from build123d import *

# Parameters (mm, degrees)
AUFSATZ_LINEAR_AUSTRAGEN1_DEPTH    = 40
DURCHGANGSLOCH_F_R_M81_D           = 8.4
DURCHGANGSLOCH_F_R_M3_51_D         = 3.7
DURCHGANGSLOCH_F_R_M82_D           = 8.4
DURCHGANGSLOCH_F_R_M82_CSINK_D     = 8.45
DURCHGANGSLOCH_F_R_M82_CSINK_ANGLE = 90
SKIZZE21_R                         = 5
SCHNITT_LINEAR_AUSTRAGEN1_DEPTH    = 12
SKIZZE22_W                         = 70
SKIZZE22_H                         = 14.633500803
SCHNITT_LINEAR_AUSTRAGEN2_DEPTH    = 20
SKIZZE23_W                         = 70
SKIZZE23_H                         = 15
SCHNITT_LINEAR_AUSTRAGEN3_DEPTH    = 26
SKIZZE25_W                         = 70
SKIZZE25_H                         = 2
SCHNITT_LINEAR_AUSTRAGEN5_DEPTH    = 26
SCHNITT_LINEAR_AUSTRAGEN6_DEPTH    = 3


with BuildPart() as part:
    # Skizze1 → Aufsatz-Linear austragen1 (new body)
    with BuildSketch(Plane.XY):
        Polygon((-85.072105864, 34.368747103), (-85.072105864, 14.368747103), (-50.072105864, 14.368747103), (-50.072105864, 28.368747103), (-65.805439197, 28.368747103), (-65.805439197, 34.368747103), align=None)
        Polygon((-50.072105864, 28.368747103), (-50.072105864, 14.368747103), (-15.072105864, 14.368747103), (-15.072105864, 34.368747103), (-34.33877253, 34.368747103), (-34.33877253, 28.368747103), align=None)
    extrude(amount=AUFSATZ_LINEAR_AUSTRAGEN1_DEPTH)

    # Durchgangsloch für M81 (through all)
    with Locations(Plane(origin=(0, 34.368747103, 0), x_dir=(1, 0, 0), z_dir=(0, 1, 0))):
        with Locations((-78.072105864, -33), (-22.072105864, -33)):
            Hole(DURCHGANGSLOCH_F_R_M81_D / 2)

    # Durchgangsloch für M3.51 (through all)
    with Locations(Plane(origin=(0, 34.368747103, 0), x_dir=(1, 0, 0), z_dir=(0, 1, 0))):
        with Locations((-78.072105864, -5), (-78.072105864, -20), (-22.072105864, -20), (-22.072105864, -5)):
            Hole(DURCHGANGSLOCH_F_R_M3_51_D / 2)

    # Durchgangsloch für M82 (through all)
    with Locations(Plane(origin=(0, 14.368747103, 0), x_dir=(-1, 0, 0), z_dir=(0, -1, 0))):
        with Locations((50.072105864, -33)):
            CounterSinkHole(DURCHGANGSLOCH_F_R_M82_D / 2, DURCHGANGSLOCH_F_R_M82_CSINK_D / 2, counter_sink_angle=DURCHGANGSLOCH_F_R_M82_CSINK_ANGLE)

    # Skizze21 → Schnitt-Linear austragen1 (cut)
    with BuildSketch(Plane(origin=(0, 28.368747103, 0), x_dir=(1, 0, 0), z_dir=(0, 1, 0))):
        with Locations((-50.072105864, -33)):
            Circle(SKIZZE21_R)
    extrude(amount=-SCHNITT_LINEAR_AUSTRAGEN1_DEPTH, mode=Mode.SUBTRACT)

    # Skizze22 → Schnitt-Linear austragen2 (cut)
    with BuildSketch(Plane(origin=(0, 34.368747103, 0), x_dir=(1, 0, 0), z_dir=(0, 1, 0))):
        with Locations((-50.072105864, -32.683249598)):
            Rectangle(SKIZZE22_W, SKIZZE22_H)
    extrude(amount=-SCHNITT_LINEAR_AUSTRAGEN2_DEPTH, mode=Mode.SUBTRACT)

    # Skizze23 → Schnitt-Linear austragen3 (cut)
    with BuildSketch(Plane(origin=(0, 0, 0), x_dir=(-1, 0, 0), z_dir=(0, 0, -1))):
        with Locations((50.072105864, 26.868747103)):
            Rectangle(SKIZZE23_W, SKIZZE23_H)
    extrude(amount=-SCHNITT_LINEAR_AUSTRAGEN3_DEPTH, mode=Mode.SUBTRACT)

    # Skizze25 → Schnitt-Linear austragen5 (cut)
    with BuildSketch(Plane.XY.offset(25.366499197)):
        with Locations((-50.072105864, 15.368747103)):
            Rectangle(SKIZZE25_W, SKIZZE25_H)
    extrude(amount=-SCHNITT_LINEAR_AUSTRAGEN5_DEPTH, mode=Mode.SUBTRACT)

    # Skizze26 → Schnitt-Linear austragen6 (cut)
    with BuildSketch(Plane.XZ.offset(-16.368747103)):
        Polygon((-40.072105864, 0), (-50.072105864, 16), (-60.072105864, 0), align=None)
    extrude(amount=-SCHNITT_LINEAR_AUSTRAGEN6_DEPTH, mode=Mode.SUBTRACT)


solid = part.part
Check sheet for the modelled part. Datum: model origin and axes. Units: mm. A direction names the side the tool comes from. Coordinates: 2 decimals unless noted, no trailing zeros. Loops run counter-clockwise (first coordinate to the right, second up) from the corner with the lowest first, then second, coordinate; pieces in that order, holes last. Notation, with made-up numbers: (9.25, 66.25) -> (57.25, 66.25) arc R14 cw to (57.25, 77.25) -> close; hole circle Ø9 at (76.25, -3.75). An arc over 180 degrees is marked (long way). Answer in a Markdown table with one row per item.
1. Release check for a two-part mould opening along Z. For faces 3 (the face through (-45.002, 17.848, 7.888)), 4 (the face through (-21.831, 17.848, 18.166)), 5 (the face through (-50, 19.369, 18)) record: released by +Z, released by -Z, zero draft, split by the parting line, or undercut.
Check values:
| item | result |
|---|---|
| face 3 | released by -Z |
| face 4 | undercut |
| face 5 | zero draft |
2. Sectioned sample at C-C, the plane y = 17.45. Record the boundary of the cut face in (x, z).
Check values:
| item | result |
|---|---|
| outline | (-85.07, 0) -> (-60.07, 0) -> (-50.07, 16) -> (-40.07, 0) -> (-15.07, 0) -> (-15.07, 25.37) -> (-85.07, 25.37) -> close; hole circle Ø3.7 at (-78.07, 5); hole circle Ø3.7 at (-78.07, 20); hole circle Ø3.7 at (-22.07, 5); hole circle Ø3.7 at (-22.07, 20) |
3. Sectioned sample at D-D, the plane z = 5. Record the boundary of the cut face in (x, y), then the cut area to 3 significant figures.
Check values:
| item | result |
|---|---|
| outline | (-85.07, 16.37) -> (-79.92, 16.37) -> (-79.92, 19.37) -> (-85.07, 19.37) -> close; (-76.22, 16.37) -> (-56.95, 16.37) -> (-56.95, 19.37) -> (-76.22, 19.37) -> close; (-43.2, 16.37) -> (-23.92, 16.37) -> (-23.92, 19.37) -> (-43.2, 19.37) -> close; (-20.22, 16.37) -> (-15.07, 16.37) -> (-15.07, 19.37) -> (-20.22, 19.37) -> close |
| area | 147 mm2 |
4. Material ranges on line 1 along X through (y, z) = (18.25, 20); line 2 along X through (y, z) = (16.55, 4.75); line 3 along Z through (x, y) = (-23, 18.1), recorded low to high. Write a range as [from, to].
Check values:
| item | result |
|---|---|
| line 1 | x = [-85.07, -79.92], [-76.22, -23.92], [-20.22, -15.07] |
| line 2 | x = [-85.07, -79.91], [-76.24, -57.1], [-43.04, -23.91], [-20.24, -15.07] |
| line 3 | z = [0, 3.4], [6.6, 18.4], [21.6, 25.37] |
5. Sectioned sample at B-B, the plane z = 8.5. Record the boundary of the cut face in (x, y), then the cut area to 3 significant figures.
Check values:
| item | result |
|---|---|
| outline | (-85.07, 16.37) -> (-54.76, 16.37) -> (-54.76, 19.37) -> (-85.07, 19.37) -> close; (-45.38, 16.37) -> (-15.07, 16.37) -> (-15.07, 19.37) -> (-45.38, 19.37) -> close |
| area | 182 mm2 |
6. Go/stop test with a flat-tipped pin: pin 1 (1.5 mm diameter, centred on x = -42, y = 17.5, fed in from -Z). Record where the tip stops, or that it passes through.
Check values:
| item | result |
|---|---|
| pin 1 | stops at z = 1.88 |
7. Access from +Z, -Z, +X, -X, +Y, -Y to the whole of each face (thin tool, end or side, straight path). Record for faces 1 (the face through (-85.072, 18, 13)), 2 (the face through (-55.002, 17.848, 8.112)).
Check values:
| item | result |
|---|---|
| face 1 | +Z, -Z, -X, +Y, -Y |
| face 2 | -Z, +Y, -Y |
8. Sectioned sample at A-A, the plane z = 20. Record the boundary of the cut face in (x, y).
Check values:
| item | result |
|---|---|
| outline | (-85.07, 16.37) -> (-79.92, 16.37) -> (-79.92, 19.37) -> (-85.07, 19.37) -> close; (-76.22, 16.37) -> (-23.92, 16.37) -> (-23.92, 19.37) -> (-76.22, 19.37) -> close; (-20.22, 16.37) -> (-15.07, 16.37) -> (-15.07, 19.37) -> (-20.22, 19.37) -> close |
